Input: part model. Units: mm. Frame: model coordinates. Face numbers are marked on the shaded views. A direction names the side the tool comes from. Coordinates: 2 decimals unless noted, no trailing zeros. Write each loop counter-clockwise with the first axis right and the second up, starting at its lowest first coordinate (ties: lowest second). Pieces come first, ordered by that corner, then holes.
1) Draft query along Y for the marked faces 6, 7 and 8. Return one class per face: pulls with the +Y half, pulls with the -Y half, needs draft (parallel to the pull), parting line crosses it, or undercut.
2) Set-up query: the marked faces 1, 2, 3, 4 and 5. Return all of +Z, -Z, +X, -X, +Y, -Y with unobstructed straight access to the full face (end or side cutting, diameter ignored); none if empty.
3) Line query: L1, parallel to Y at x = -6, z = 11; L2, parallel to Z at x = -7.5, y = -8.5; L3, parallel to Z at x = 2, y = -23.25. Output: solid intervals per line, ascending.
4) Section query C-C (y = -17.25). Output: boundary loops of the cut face in (x, z).
5) Pin query (flat end, axial travel): pin 1 Ø11 at (x, z) = (2, 16) entering from +Y; pin 2 Ø4 at (y, z) = (-12.5, -0.5) entering from -X; pin 3 Ø5 at (x, z) = (-2.5, 13) entering from -Y. Return the tip coordinate at first contact, or that it passes through.
6) Section query D-D (z = -7). Output: boundary loops of the cut face in (x, y).
7) Section query A-A (y = -12.5). State how many separate pieces and enclosed holes the cut face has, then the cut area to 3 significant figures.
8) Section query B-B (x = 7.5). Output: boundary loops of the cut face in (y, z).
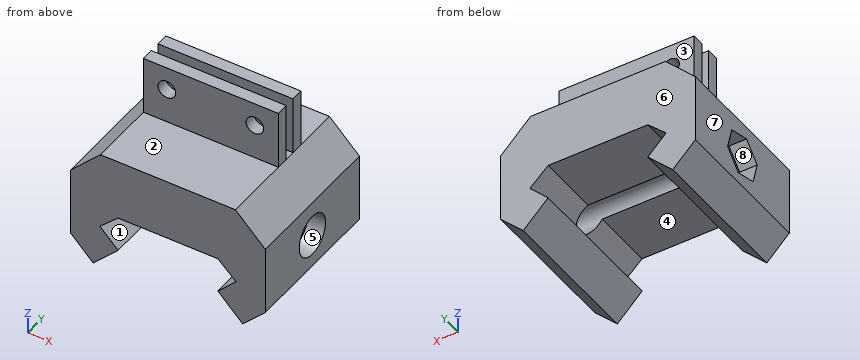
from build123d import *

# Parameters (mm, degrees)
F1_DEPTH  = 25
F2_W      = 7.596032
F2_H      = 21.10009
F2_W_2    = 10.268714
F2_H_2    = 30.102797
F3_DEPTH  = 25
F4_R      = 2
F5_DEPTH  = 35
F6_R      = 3.5
F7_DEPTH  = 3
F9_DEPTH  = 3
F10_W     = 23
F10_H     = 6
F11_DEPTH = 10
F12_W     = 23
F12_H     = 1.8
F13_DEPTH = 10
F14_R     = 1.5
F15_DEPTH = 25


with BuildPart() as f1:
    # F0 (on Front) → F1 (new body)
    with BuildSketch(Plane.XZ):
        Polygon((-11.604762, -2.895238), (-8.5, 0), (8.5, 0), (11.604762, -2.895238), (8.5, -6), (12.742641, -10.242641), (22.464761, -0.520521), (11.5, 10.44424), (-11.5, 10.44424), (-22.464761, -0.520521), (-12.742641, -10.242641), (-8.5, -6), align=None)
    extrude(amount=F1_DEPTH)

    # F2 (on face) → F3 (cut)
    with BuildSketch(Plane.XZ.offset(25)):
        with Locations((-20.402778, -0.557668)):
            Rectangle(F2_W, F2_H)
        with Locations((21.739119, -1.542339)):
            Rectangle(F2_W_2, F2_H_2)
    extrude(amount=-F3_DEPTH, mode=Mode.SUBTRACT)

    # F4 (on face) → F5 (cut)
    with BuildSketch(Plane.YZ.offset(16.604762)):
        with Locations((-12.5, -0.695238)):
            Circle(F4_R)
    extrude(amount=-F5_DEPTH, mode=Mode.SUBTRACT)

    # F6 (on face) → F7 (cut)
    with BuildSketch(Plane.YZ.offset(16.604762)):
        with Locations((-12.5, -0.695238)):
            Circle(F6_R)
    extrude(amount=-F7_DEPTH, mode=Mode.SUBTRACT)

    # F8 (on face) → F9 (cut)
    with BuildSketch(Plane(origin=(-16.604762, 0, 0), x_dir=(0, -1, 0), z_dir=(-1, 0, 0))):
        Polygon((15.321942, -3.588329), (16.416462, 0.30209), (13.59452, 3.195181), (9.678058, 2.197854), (8.583538, -1.692565), (11.40548, -4.585657), align=None)
    extrude(amount=-F9_DEPTH, mode=Mode.SUBTRACT)

    # F10 (on face) → F11 (join)
    with BuildSketch(Plane.XY.offset(10.44424)):
        with Locations((0, -10.598838)):
            Rectangle(F10_W, F10_H)
    extrude(amount=F11_DEPTH)

    # F12 (on face) → F13 (cut)
    with BuildSketch(Plane.XY.offset(20.44424)):
        with Locations((0, -10.598838)):
            Rectangle(F12_W, F12_H)
    extrude(amount=-F13_DEPTH, mode=Mode.SUBTRACT)

    # F14 (on face) → F15 (cut)
    with BuildSketch(Plane(origin=(0, -7.598838, 0), x_dir=(-1, 0, 0), z_dir=(0, 1, 0))):
        with Locations((-7.5, 16.44424)):
            Circle(F14_R)
        with Locations((7.5, 16.44424)):
            Circle(F14_R)
    extrude(amount=-F15_DEPTH, mode=Mode.SUBTRACT)


solid = f1.part
Answer:
1. face 6: pulls with the +Y half
1. face 7: needs draft
1. face 8: undercut
2. face 1: +Y, -Y
2. face 2: +Z, +X, -X, -Y
2. face 3: +Z, +X, -X, +Y
2. face 4: -Z, +Y, -Y
2. face 5: +X
3. L1: y = -13.6 to -11.5, -9.7 to -7.6
3. L2: z = 0 to 14.94, 17.94 to 20.44
3. L3: z = 0 to 10.44
4. outline: (-16.6, -6.38) - (-12.74, -10.24) - (-8.5, -6) - (-11.6, -2.9) - (-8.5, 0) - (8.5, 0) - (11.6, -2.9) - (8.5, -6) - (12.74, -10.24) - (16.6, -6.38) - (16.6, 5.34) - (11.5, 10.44) - (-11.5, 10.44) - (-16.6, 5.34) - close
5. pin 1: stops at y = -7.6
5. pin 2: stops at x = -13.6
5. pin 3: stops at y = -13.6
6. outline: (-15.99, -25) - (-9.5, -25) - (-9.5, 0) - (-15.99, 0) - close; (9.5, -25) - (15.99, -25) - (15.99, 0) - (9.5, 0) - close
7. separate pieces: 3
7. enclosed holes: 2
7. area: 553 mm2
8. outline: (-25, 0) - (-14.38, 0) arc R2 cw to (-10.62, 0) - (0, 0) - (0, 10.44) - (-7.6, 10.44) - (-7.6, 14.94) - (-9.7, 14.94) - (-9.7, 10.44) - (-11.5, 10.44) - (-11.5, 14.94) - (-13.6, 14.94) - (-13.6, 10.44) - (-25, 10.44) - close; (-13.6, 17.94) - (-11.5, 17.94) - (-11.5, 20.44) - (-13.6, 20.44) - close; (-9.7, 17.94) - (-7.6, 17.94) - (-7.6, 20.44) - (-9.7, 20.44) - close
